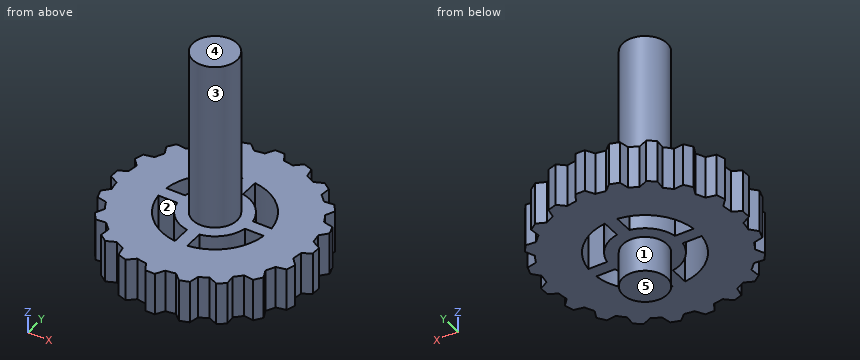
```python
from build123d import *

# Parameters (mm, degrees)
DODANIE_WYCI_GNI_CIE2_DEPTH = 2.4
SZKIC2_R                    = 1.25
DODANIE_WYCI_GNI_CIE3_DEPTH = 2
DODANIE_WYCI_GNI_CIE4_START = 9.5
SZKIC3_R                    = 1.25
DODANIE_WYCI_GNI_CIE4_DEPTH = 9.5
WYTNIJ_WYCI_GNI_CIE1_DEPTH  = 9.5


with BuildPart() as part:
    # Szkic1 → Dodanie-wyciągnięcie2 (new body)
    with BuildSketch(Plane.XY):
        with BuildLine():
            Line((2.133245608, 4.797057762), (2.016205978, 5.347685932))
            Line((2.016205978, 5.347685932), (1.512146024, 5.511464939))
            Line((1.512146024, 5.511464939), (1.093807857, 5.134791561))
            ThreePointArc((1.093807857, 5.134791561), (0.821280941, 5.185363788), (0.546464765, 5.22148219))
            Line((0.546464765, 5.22148219), (0.265, 5.708993464))
            Line((0.265, 5.708993464), (-0.265, 5.708993464))
            Line((-0.265, 5.708993464), (-0.546464765, 5.22148219))
            ThreePointArc((-0.546464765, 5.22148219), (-0.821280941, 5.185363788), (-1.093807857, 5.134791561))
            Line((-1.093807857, 5.134791561), (-1.512146024, 5.511464939))
            Line((-1.512146024, 5.511464939), (-2.016205978, 5.347685932))
            Line((-2.016205978, 5.347685932), (-2.133245608, 4.797057762))
            ThreePointArc((-2.133245608, 4.797057762), (-2.383450124, 4.677784252), (-2.627010944, 4.545471757))
            Line((-2.627010944, 4.545471757), (-3.14127266, 4.774435825))
            Line((-3.14127266, 4.774435825), (-3.570051667, 4.462909641))
            Line((-3.570051667, 4.462909641), (-3.511209508, 3.903063898))
            ThreePointArc((-3.511209508, 3.903063898), (-3.712310601, 3.712310601), (-3.903063898, 3.511209508))
            Line((-3.903063898, 3.511209508), (-4.462909641, 3.570051667))
            Line((-4.462909641, 3.570051667), (-4.774435825, 3.14127266))
            Line((-4.774435825, 3.14127266), (-4.545471757, 2.627010944))
            ThreePointArc((-4.545471757, 2.627010944), (-4.677784252, 2.383450124), (-4.797057762, 2.133245608))
            Line((-4.797057762, 2.133245608), (-5.347685932, 2.016205978))
            Line((-5.347685932, 2.016205978), (-5.511464939, 1.512146024))
            Line((-5.511464939, 1.512146024), (-5.134791561, 1.093807857))
            ThreePointArc((-5.134791561, 1.093807857), (-5.185363788, 0.821280941), (-5.22148219, 0.546464765))
            Line((-5.22148219, 0.546464765), (-5.708993464, 0.265))
            Line((-5.708993464, 0.265), (-5.708993464, -0.265))
            Line((-5.708993464, -0.265), (-5.22148219, -0.546464765))
            ThreePointArc((-5.22148219, -0.546464765), (-5.185363788, -0.821280941), (-5.134791561, -1.093807857))
            Line((-5.134791561, -1.093807857), (-5.511464939, -1.512146024))
            Line((-5.511464939, -1.512146024), (-5.347685932, -2.016205978))
            Line((-5.347685932, -2.016205978), (-4.797057762, -2.133245608))
            ThreePointArc((-4.797057762, -2.133245608), (-4.677784252, -2.383450124), (-4.545471757, -2.627010944))
            Line((-4.545471757, -2.627010944), (-4.774435825, -3.14127266))
            Line((-4.774435825, -3.14127266), (-4.462909641, -3.570051667))
            Line((-4.462909641, -3.570051667), (-3.903063898, -3.511209508))
            ThreePointArc((-3.903063898, -3.511209508), (-3.712310601, -3.712310601), (-3.511209508, -3.903063898))
            Line((-3.511209508, -3.903063898), (-3.570051667, -4.462909641))
            Line((-3.570051667, -4.462909641), (-3.14127266, -4.774435825))
            Line((-3.14127266, -4.774435825), (-2.627010944, -4.545471757))
            ThreePointArc((-2.627010944, -4.545471757), (-2.383450124, -4.677784252), (-2.133245608, -4.797057762))
            Line((-2.133245608, -4.797057762), (-2.016205978, -5.347685932))
            Line((-2.016205978, -5.347685932), (-1.512146024, -5.511464939))
            Line((-1.512146024, -5.511464939), (-1.093807857, -5.134791561))
            ThreePointArc((-1.093807857, -5.134791561), (-0.821280941, -5.185363788), (-0.546464765, -5.22148219))
            Line((-0.546464765, -5.22148219), (-0.265, -5.708993464))
            Line((-0.265, -5.708993464), (0.265, -5.708993464))
            Line((0.265, -5.708993464), (0.546464765, -5.22148219))
            ThreePointArc((0.546464765, -5.22148219), (0.821280941, -5.185363788), (1.093807857, -5.134791561))
            Line((1.093807857, -5.134791561), (1.512146024, -5.511464939))
            Line((1.512146024, -5.511464939), (2.016205978, -5.347685932))
            Line((2.016205978, -5.347685932), (2.133245608, -4.797057762))
            ThreePointArc((2.133245608, -4.797057762), (2.383450124, -4.677784252), (2.627010944, -4.545471757))
            Line((2.627010944, -4.545471757), (3.14127266, -4.774435825))
            Line((3.14127266, -4.774435825), (3.570051667, -4.462909641))
            Line((3.570051667, -4.462909641), (3.511209508, -3.903063898))
            ThreePointArc((3.511209508, -3.903063898), (3.712310601, -3.712310601), (3.903063898, -3.511209508))
            Line((3.903063898, -3.511209508), (4.462909641, -3.570051667))
            Line((4.462909641, -3.570051667), (4.774435825, -3.14127266))
            Line((4.774435825, -3.14127266), (4.545471757, -2.627010944))
            ThreePointArc((4.545471757, -2.627010944), (4.677784252, -2.383450124), (4.797057762, -2.133245608))
            Line((4.797057762, -2.133245608), (5.347685932, -2.016205978))
            Line((5.347685932, -2.016205978), (5.511464939, -1.512146024))
            Line((5.511464939, -1.512146024), (5.134791561, -1.093807857))
            ThreePointArc((5.134791561, -1.093807857), (5.185363788, -0.821280941), (5.22148219, -0.546464765))
            Line((5.22148219, -0.546464765), (5.708993464, -0.265))
            Line((5.708993464, -0.265), (5.708993464, 0.265))
            Line((5.708993464, 0.265), (5.22148219, 0.546464765))
            ThreePointArc((5.22148219, 0.546464765), (5.185363788, 0.821280941), (5.134791561, 1.093807857))
            Line((5.134791561, 1.093807857), (5.511464939, 1.512146024))
            Line((5.511464939, 1.512146024), (5.347685932, 2.016205978))
            Line((5.347685932, 2.016205978), (4.797057762, 2.133245608))
            ThreePointArc((4.797057762, 2.133245608), (4.677784252, 2.383450124), (4.545471757, 2.627010944))
            Line((4.545471757, 2.627010944), (4.774435825, 3.14127266))
            Line((4.774435825, 3.14127266), (4.462909641, 3.570051667))
            Line((4.462909641, 3.570051667), (3.903063898, 3.511209508))
            ThreePointArc((3.903063898, 3.511209508), (3.712310601, 3.712310601), (3.511209508, 3.903063898))
            Line((3.511209508, 3.903063898), (3.570051667, 4.462909641))
            Line((3.570051667, 4.462909641), (3.14127266, 4.774435825))
            Line((3.14127266, 4.774435825), (2.627010944, 4.545471757))
            ThreePointArc((2.627010944, 4.545471757), (2.383450124, 4.677784252), (2.133245608, 4.797057762))
        make_face()
    extrude(amount=DODANIE_WYCI_GNI_CIE2_DEPTH)

    # Szkic2 → Dodanie-wyciągnięcie3 (add)
    with BuildSketch(Plane(origin=(0, 0, 0), x_dir=(-1, 0, 0), z_dir=(0, 0, -1))):
        with Locations(Location((0, 0, 0), (0, 0, 180))):
            Circle(SZKIC2_R)
    extrude(amount=DODANIE_WYCI_GNI_CIE3_DEPTH)

    # Szkic3 → Dodanie-wyciągnięcie4 (add)
    with BuildSketch(Plane.XY.offset(2.4).offset(DODANIE_WYCI_GNI_CIE4_START)):
        Circle(SZKIC3_R)
    extrude(amount=-DODANIE_WYCI_GNI_CIE4_DEPTH)

    # Szkic4 → Wytnij-wyciągnięcie1 (cut)
    with BuildSketch(Plane(origin=(0, 0, 0), x_dir=(-1, 0, 0), z_dir=(0, 0, -1))):
        with BuildLine():
            Line((-2.979513383, 0.35), (-1.918332609, 0.35))
            ThreePointArc((-1.918332609, 0.35), (-1.378858223, 1.378858223), (-0.35, 1.918332609))
            Line((-0.35, 1.918332609), (-0.35, 2.979513383))
            ThreePointArc((-0.35, 2.979513383), (-2.121320344, 2.121320344), (-2.979513383, 0.35))
        make_face()
        with BuildLine():
            Line((-2.979513383, -0.35), (-1.918332609, -0.35))
            ThreePointArc((-1.918332609, -0.35), (-1.378858223, -1.378858223), (-0.35, -1.918332609))
            Line((-0.35, -1.918332609), (-0.35, -2.979513383))
            ThreePointArc((-0.35, -2.979513383), (-2.121320344, -2.121320344), (-2.979513383, -0.35))
        make_face()
        with BuildLine():
            Line((1.918332609, 0.35), (2.979513383, 0.35))
            ThreePointArc((2.979513383, 0.35), (2.121320344, 2.121320344), (0.35, 2.979513383))
            Line((0.35, 2.979513383), (0.35, 1.918332609))
            ThreePointArc((0.35, 1.918332609), (1.378858223, 1.378858223), (1.918332609, 0.35))
        make_face()
        with BuildLine():
            Line((1.918332609, -0.35), (2.979513383, -0.35))
            ThreePointArc((2.979513383, -0.35), (2.121320344, -2.121320344), (0.35, -2.979513383))
            Line((0.35, -2.979513383), (0.35, -1.918332609))
            ThreePointArc((0.35, -1.918332609), (1.378858223, -1.378858223), (1.918332609, -0.35))
        make_face()
    extrude(amount=-WYTNIJ_WYCI_GNI_CIE1_DEPTH, mode=Mode.SUBTRACT)


solid = part.part
```
Geometry: final body of the model. Coordinates: model frame, mm. Face numbers are marked on the shaded views. A direction names the side the tool comes from. Round coordinates to 2 decimals unless told otherwise and drop trailing zeros. Loops run counter-clockwise (first coordinate to the right, second up) from the corner with the lowest first, then second, coordinate; pieces in that order, holes last. Notation, with made-up numbers: (-12.5, 89) -> (39.5, 89) arc R6 cw to (39.5, 98) -> close; hole circle Ø3 at (40, 72.5). An arc over 180 degrees is marked (long way). Write each question's results on one line, items separated by ' | '.
Item 1: Set-up query: the marked faces 1, 2, 3, 4 and 5. Return all of +Z, -Z, +X, -X, +Y, -Y with unobstructed straight access to the full face (end or side cutting, diameter ignored); none if empty.
Answers below:
face 1: -Z | face 2: +Z, -Z | face 3: +Z | face 4: +Z, +X, -X, +Y, -Y | face 5: -Z, +X, -X, +Y, -Y
Item 2: Line query: probe 1 along Z at (x, y) = (-1.75, -0.5); probe 2 along Y at (x, z) = (0.5, 1.5); probe 3 along X at (y, z) = (-2.25, 2). Output: solid intervals per line, ascending. Write a range as [from, to].
Answers below:
probe 1: z = [0, 2.4] | probe 2: y = [-5.3, -2.96], [-1.88, 1.88], [2.96, 5.3] | probe 3: x = [-4.74, -1.98], [-0.35, 0.35], [1.98, 4.74]
Item 3: Cut plane C-C on z = 1.25. State how many separate pieces and enclosed holes the cut face has, and give its area (3 significant figures).
Answers below:
separate pieces: 1 | enclosed holes: 4 | area: 80.7 mm²
Item 4: Cut plane D-D on z = 3. Return the cut outline in (x, y).
Answers below:
outline: circle Ø2.5 at (0, 0)
Item 5: Cut plane B-B on y = 0. Return the cut outline in (x, z), and give its area (3 significant figures).
Answers below:
outline: (-5.71, 0) -> (-1.25, 0) -> (-1.25, -2) -> (1.25, -2) -> (1.25, 0) -> (5.71, 0) -> (5.71, 2.4) -> (1.25, 2.4) -> (1.25, 11.9) -> (-1.25, 11.9) -> (-1.25, 2.4) -> (-5.71, 2.4) -> close | area: 56.2 mm²
Item 6: Cut plane A-A on x = 0.75. Return the cut outline in (y, z).
Answers below:
outline: (-5.2, 0) -> (-2.9, 0) -> (-2.9, 2.4) -> (-5.2, 2.4) -> close; (-1.8, 0) -> (-1, 0) -> (-1, -2) -> (1, -2) -> (1, 0) -> (1.8, 0) -> (1.8, 2.4) -> (1, 2.4) -> (1, 11.9) -> (-1, 11.9) -> (-1, 2.4) -> (-1.8, 2.4) -> close; (2.9, 0) -> (5.2, 0) -> (5.2, 2.4) -> (2.9, 2.4) -> close
Item 7: Pin query (flat end, axial travel): pin 1 Ø1.5 at (x, y) = (-3, 3.5) entering from +Z; pin 2 Ø2 at (y, z) = (-4, 9) entering from +X; pin 3 Ø0.5 at (x, z) = (-2.5, 1) entering from +Y; pin 4 Ø0.5 at (y, z) = (2.5, 1.5) entering from -X. Return the tip coordinate at first contact, or that it passes through.
Answers below:
pin 1: stops at z = 2.4 | pin 2: passes through | pin 3: stops at y = 4.74 | pin 4: stops at x = -4.74
